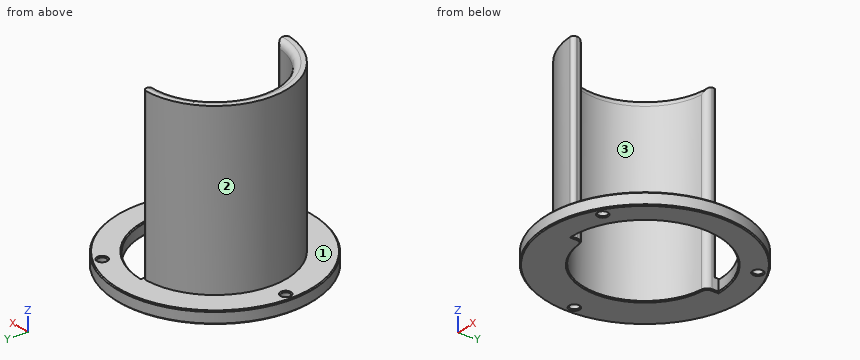
from build123d import *

# Parameters (mm, degrees)
SKETCH_R     = 40.2
SKETCH_R_2   = 25
PAD_DEPTH    = 5
PAD001_DEPTH = 74
POCKET_DEPTH = 5
FILLET_R     = 1.5
FILLET001_R  = 2.6
SKETCH003_R  = 1.8
HOLE_DEPTH   = 5
CHAMFER_SIZE = 0.4


with BuildPart() as part:
    # Sketch → Pad (new body)
    with BuildSketch(Plane.XY):
        Circle(SKETCH_R)
        Circle(SKETCH_R_2, mode=Mode.SUBTRACT)
    extrude(amount=PAD_DEPTH)

    # Sketch001 → Pad001 (join)
    with BuildSketch(Plane.XY):
        with BuildLine():
            ThreePointArc((0, 29.5), (-29.5, 0), (0, -29.5))
            Line((0, -25), (0, -29.5))
            ThreePointArc((0, 25), (-25, 0), (0, -25))
            Line((0, 29.5), (0, 25))
        make_face()
    extrude(amount=PAD001_DEPTH)

    # Sketch002 → Pocket (cut)
    with BuildSketch(Plane.XY):
        with BuildLine():
            ThreePointArc((0, -30), (30, 0), (0, 30))
            Line((0, 30), (0, 25))
            ThreePointArc((0, -25), (25, 0), (0, 25))
            Line((0, -25), (0, -30))
        make_face()
    extrude(amount=POCKET_DEPTH, mode=Mode.SUBTRACT)

    # Fillet
    fillet_edges = [part.edges().sort_by_distance(p)[0] for p in [
        (0, -29.5, 39.5),
        (0, 29.5, 39.5),
    ]]
    fillet(fillet_edges, radius=FILLET_R)

    # Fillet001
    fillet001_edges = [part.edges().sort_by_distance(p)[0] for p in [
        (-25, 0, 74),
        (0, -25, 39.5),
        (0, 25, 39.5),
    ]]
    fillet(fillet001_edges, radius=FILLET001_R)

    # Sketch003 → Hole (cut)
    with BuildSketch(Plane.XY):
        with Locations((-36.6, 0)):
            Circle(SKETCH003_R)
        with Locations((18.3, 31.69653)):
            Circle(SKETCH003_R)
        with Locations((18.3, -31.69653)):
            Circle(SKETCH003_R)
    extrude(amount=HOLE_DEPTH, mode=Mode.SUBTRACT)

    # Chamfer
    chamfer_edges = [part.edges().sort_by_distance(p)[0] for p in [
        (-40.2, 0, 0),
        (20.1, -31.69653, 0),
        (-34.8, 0, 0),
        (20.1, 31.69653, 0),
        (30, 0, 0),
        (0, -29.75, 0),
        (0, -28.488632, 0),
        (-0.676876, -25.727522, 0),
        (-25, 0, 0),
        (0, 29.75, 0),
        (0, 28.488632, 0),
        (-0.676876, 25.727522, 0),
        (-40.2, 0, 5),
        (-34.8, 0, 5),
        (20.1, 31.69653, 5),
        (20.1, -31.69653, 5),
        (30, 0, 5),
    ]]
    chamfer(chamfer_edges, length=CHAMFER_SIZE)


solid = part.part
Design review of the part built by this model. Coordinates are the model's own, in mm. Face numbers are marked on the shaded views. Coordinates: 2 decimals unless noted, no trailing zeros. Loops run counter-clockwise (first coordinate to the right, second up) from the corner with the lowest first, then second, coordinate; pieces in that order, holes last. Notation, with made-up numbers: (71, -25.75) -> (89, -25.75) arc R19 cw to (89, -17.75) -> close; hole circle Ø4 at (53.25, 27.5). An arc over 180 degrees is marked (long way). Use a Markdown table: item, result. Add a question column.
Item 1: Wall thickness on L1, parallel to Y at x = 18.3, z = 2.75; L2, parallel to Z at x = -30, y = 23; L3, parallel to Y at x = -11, z = 67: over which ranges is each line inside the solid? List them lowest first. Write a range as from..to.
Item 2: We need section B-B, the plane y = 0. Write out the cut boundary in (x, z), and give its area (3 significant figures).
Item 3: We need section A-A, the plane z = 52. Write out the cut boundary in (x, y).
Item 4: We need section C-C, the plane x = 18.3. Count the separate pieces of the cut face and the enclosed holes in it, and give its area (3 significant figures).
Item 5: Clearance check with flat-ended pins moving along their axes: P1, Ø8, axis at y = -17, z = 45, coming from the -X side; P2, Ø6, axis at x = -36.6, y = 0, coming from the +Z side; P3, Ø5, axis at x = -5.5, z = 63.5, coming from the +Y side; P4, Ø6, axis at x = 18.3, y = 31.7, coming from the -Z side. State where each tip first meets the part, or that it passes through.
Item 6: The part is to be moulded in two halves that separate along Y. For the marked faces 1, 2 and 3, say which applies: +Y half, -Y half, draft (parallel to the pull), parting line (faces both ways), or undercut.
Numbers:
| question | item | result |
|---|---|---|
| 1 | L1 | y = -35.79..-33.5, -29.9..-23.77, 23.77..29.9, 33.5..35.79 |
| 1 | L2 | z = 0..5 |
| 1 | L3 | y = -27.37..-22.45, 22.45..27.37 |
| 2 | outline | (-40.2, 0.4) -> (-39.8, 0) -> (-38.8, 0) -> (-38.4, 0.4) -> (-38.4, 4.6) -> (-38.8, 5) -> (-39.8, 5) -> (-40.2, 4.6) -> close; (-34.8, 0.4) -> (-34.4, 0) -> (-25.4, 0) -> (-25, 0.4) -> (-25, 71.4) arc R2.6 ccw to (-27.6, 74) -> (-29.5, 74) -> (-29.5, 5) -> (-34.4, 5) -> (-34.8, 4.6) -> close; (30, 0.4) -> (30.4, 0) -> (39.8, 0) -> (40.2, 0.4) -> (40.2, 4.6) -> (39.8, 5) -> (30.4, 5) -> (30, 4.6) -> close |
| 2 | area | 417 mm^2 |
| 3 | outline | (-2.36, -24.89) arc R25 cw to (-2.36, 24.89) arc R2.6 ccw to (0, 27.48) -> (0, 27.96) arc R1.5 ccw to (-1.58, 29.46) arc R29.5 ccw to (-1.58, -29.46) arc R1.5 ccw to (0, -27.96) -> (0, -27.48) arc R2.6 ccw to start |
| 4 | separate pieces | 4 |
| 4 | enclosed holes | 0 |
| 4 | area | 82.8 mm^2 |
| 5 | P1 | stops at x = -26.48 |
| 5 | P2 | stops at z = 5 |
| 5 | P3 | stops at y = 29.35 |
| 5 | P4 | stops at z = 0 |
| 6 | face 1 | draft |
| 6 | face 2 | parting line |
| 6 | face 3 | undercut |
